Can you work these out from the drawing? Everything is in mm from the part's minimum corner. Round coordinates to 2 decimals unless told otherwise and drop trailing zeros. Order: outer loops, then holes, each group sorted by start corner. A loop starts at its lowest first (then second) coordinate and runs counter-clockwise, first axis right, second up. Notation, with made-up numbers: (-19, -30.75) -> (-6, -30.75) arc R34 cw to (-6, 6.25) -> close; hole circle Ø8 at (61.25, -10). An arc over 180 degrees is marked (long way). One line per item, written item: value.
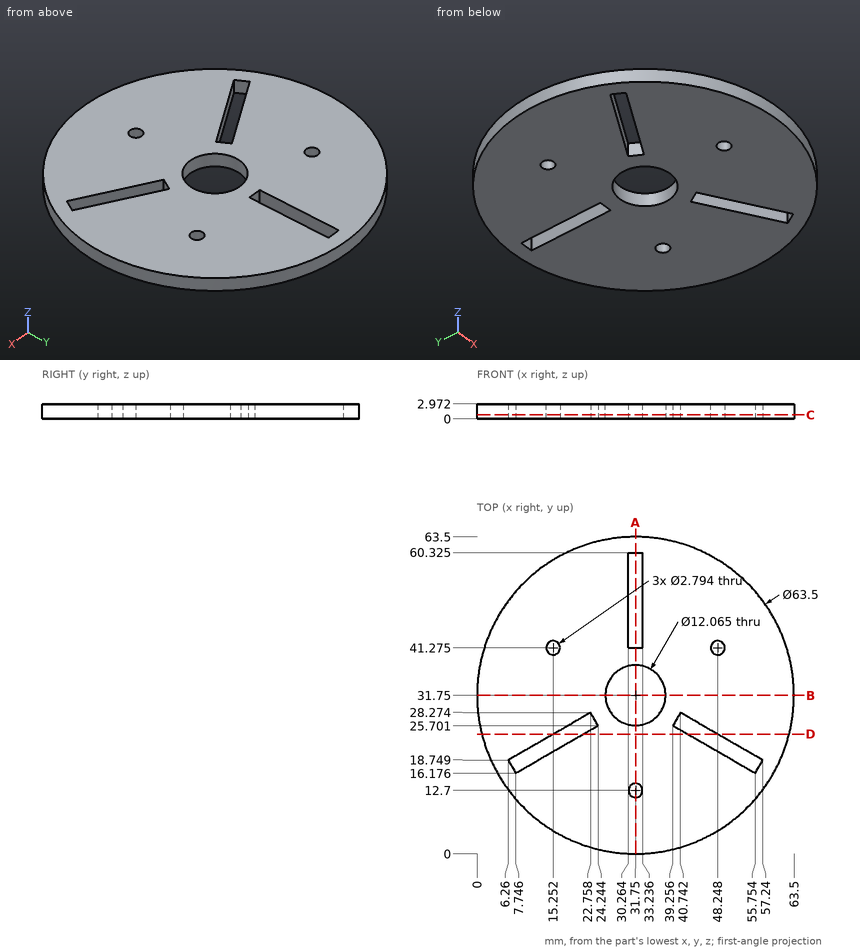
Q1. I want a section at B-B on y = 31.75. Write out the boundary of the cut face in (x, z).
Answers:
outline: (0, 0) -> (25.72, 0) -> (25.72, 2.97) -> (0, 2.97) -> close; (37.78, 0) -> (63.5, 0) -> (63.5, 2.97) -> (37.78, 2.97) -> close
Q2. I want a section at C-C on z = 0.8. Give the number of separate pieces and of enclosed holes in the cut face, then the cut area to 3 significant figures.
Answers:
separate pieces: 1
enclosed holes: 7
area: 2,860 mm2
Q3. I need wall thicknesses on line 1 along Y through (x, z) = (31.75, 1.8) (1 decimal); line 2 along X through (y, z) = (32, 1.9); line 3 along X through (y, z) = (12.7, 1.8). Which ranges of each line are inside material? Lowest first, please.
Answers:
line 1: 0 to 11.3, 14.1 to 25.7, 37.8 to 41.3, 60.3 to 63.5
line 2: 0 to 25.72, 37.78 to 63.5
line 3: 6.35 to 30.35, 33.15 to 57.15
Q4. I want a section at D-D on y = 24. Write out the boundary of the cut face in (x, z) (1 decimal), then the cut area to 3 significant figures.
Answers:
outline: (1, 0) -> (15.4, 0) -> (15.4, 3) -> (1, 3) -> close; (21.3, 0) -> (42.2, 0) -> (42.2, 3) -> (21.3, 3) -> close; (48.1, 0) -> (62.5, 0) -> (62.5, 3) -> (48.1, 3) -> close
area: 148 mm2
Q5. I want a section at A-A on x = 31.75. Write out the boundary of the cut face in (y, z) (1 decimal).
Answers:
outline: (0, 0) -> (11.3, 0) -> (11.3, 3) -> (0, 3) -> close; (14.1, 0) -> (25.7, 0) -> (25.7, 3) -> (14.1, 3) -> close; (37.8, 0) -> (41.3, 0) -> (41.3, 3) -> (37.8, 3) -> close; (60.3, 0) -> (63.5, 0) -> (63.5, 3) -> (60.3, 3) -> close
Q6. For P1, Ø0.9, axis at y = 49, z = 1.5, coming from the +X side; P2, Ø2.5, axis at x = 15.25, y = 41.28, coming from the +Z side; P3, Ø1.5, axis at x = 32, z = 1, coming from the +Y side, each with a flat end and sliding along its axis, tell me the tip position at first contact or that it passes through.
Answers:
P1: x = 58.69
P2: through
P3: y = 63.5
